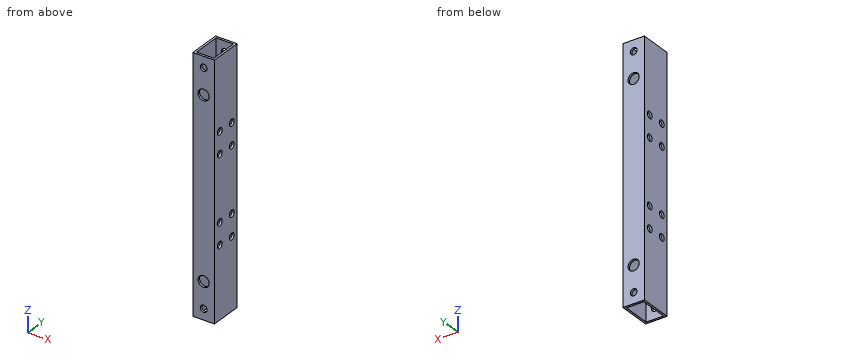
from build123d import *

# Parameters (mm, degrees)
SKETCH_1_W          = 10
SKETCH_1_H          = 15
SKETCH_1_W_2        = 8
SKETCH_1_H_2        = 13
EXTRUDE_1_DEPTH     = 116
SKETCH_2_R          = 1.575
SKETCH_2_R_2        = 2.575
CUT_EXTRUDE_1_DEPTH = 118.39250402
SKETCH_3_R          = 1.575
CUT_EXTRUDE_2_DEPTH = 118.39250402


with BuildPart() as part:
    # 草图1 → 拉伸-薄壁1 (new body)
    with BuildSketch(Plane.XY):
        with Locations((5, -7.5)):
            Rectangle(SKETCH_1_W, SKETCH_1_H)
        with Locations((5, -7.5)):
            Rectangle(SKETCH_1_W_2, SKETCH_1_H_2, mode=Mode.SUBTRACT)
    extrude(amount=EXTRUDE_1_DEPTH)

    # 草图2 → 切除-拉伸1 (cut, through all)
    with BuildSketch(Plane(origin=(0, 0, 0), x_dir=(1, 0, 0), z_dir=(0, 1, 0))):
        with Locations(Location((5, -5, 0), (0, 0, 270))):
            Circle(SKETCH_2_R)
        with Locations(Location((5, -17, 0), (0, 0, 270))):
            Circle(SKETCH_2_R_2)
        with Locations(Location((5, -99, 0), (0, 0, 270))):
            Circle(SKETCH_2_R_2)
        with Locations(Location((5, -111, 0), (0, 0, 270))):
            Circle(SKETCH_2_R)
    extrude(amount=-CUT_EXTRUDE_1_DEPTH, mode=Mode.SUBTRACT)

    # 草图3 → 切除-拉伸2 (cut, through all)
    with BuildSketch(Plane.ZY):
        with Locations(Location((33, -3.5, 0), (0, 0, 270))):
            Circle(SKETCH_3_R)
        with Locations(Location((43, -3.5, 0), (0, 0, 90))):
            Circle(SKETCH_3_R)
        with Locations(Location((43, -11.5, 0), (0, 0, 270))):
            Circle(SKETCH_3_R)
        with Locations(Location((33, -11.5, 0), (0, 0, 90))):
            Circle(SKETCH_3_R)
        with Locations(Location((83, -11.5, 0), (0, 0, 270))):
            Circle(SKETCH_3_R)
        with Locations(Location((73, -11.5, 0), (0, 0, 90))):
            Circle(SKETCH_3_R)
        with Locations(Location((73, -3.5, 0), (0, 0, 270))):
            Circle(SKETCH_3_R)
        with Locations(Location((83, -3.5, 0), (0, 0, 90))):
            Circle(SKETCH_3_R)
    extrude(amount=-CUT_EXTRUDE_2_DEPTH, mode=Mode.SUBTRACT)


solid = part.part
Source: CAD feature listing. Evaluate the final solid. Frame: model axes, mm. Round coordinates to 2 decimals unless told otherwise and drop trailing zeros. Write each loop counter-clockwise with the first axis right and the second up, starting at its lowest first coordinate (ties: lowest second). Pieces come first, ordered by that corner, then holes. Notation, with made-up numbers: (-33.75, -26.75) - (0.25, -26.75) arc R28 ccw to (0.25, -8.75) - close; hole circle Ø11 at (-5.75, 7). An arc over 180 degrees is marked (long way). Use CSV: the item, a comma, the result in double quotes. Start each with the question number.
(1) Material intervals for probe 1 along Z at (x, y) = (9.55, -3.5) (3 decimals); probe 2 along Y at (x, z) = (3.5, 55); probe 3 along X at (y, z) = (-11.25, 14.5), sorted ascending. Write a range as [from, to].
(2) Cut plane D-D, the plane z = 73. Return loops of the section in (x, y) (3 decimals).
(3) Cut plane A-A, the plane z = 17. Return loops of the section in (x, y) (3 decimals).
(4) Cut plane B-B, the plane y = -7. Return loops of the section in (x, z), and give its area (3 significant figures).
(5) Cut plane C-C, the plane z = 53.5. Return loops of the section in (x, y).
Geometry says:
1,probe 1,"[0, 31.425], [34.575, 41.425], [44.575, 71.425], [74.575, 81.425], [84.575, 116]"
1,probe 2,"[-15, -14], [-1, 0]"
1,probe 3,"[0, 1], [9, 10]"
2,outline,"(0, -15) - (10, -15) - (10, -13.075) - (9, -13.075) - (9, -14) - (1, -14) - (1, -13.075) - (0, -13.075) - close; (0, -9.925) - (1, -9.925) - (1, -5.075) - (0, -5.075) - close; (0, -1.925) - (1, -1.925) - (1, -1) - (9, -1) - (9, -1.925) - (10, -1.925) - (10, 0) - (0, 0) - close; (9, -9.925) - (10, -9.925) - (10, -5.075) - (9, -5.075) - close"
3,outline,"(0, -15) - (2.425, -15) - (2.425, -14) - (1, -14) - (1, -1) - (2.425, -1) - (2.425, 0) - (0, 0) - close; (7.575, -15) - (10, -15) - (10, 0) - (7.575, 0) - (7.575, -1) - (9, -1) - (9, -14) - (7.575, -14) - close"
4,outline,"(0, 0) - (1, 0) - (1, 116) - (0, 116) - close; (9, 0) - (10, 0) - (10, 116) - (9, 116) - close"
4,area,"232 mm²"
5,outline,"(0, -15) - (10, -15) - (10, 0) - (0, 0) - close; hole (1, -14) - (9, -14) - (9, -1) - (1, -1) - close"
